Input: part model. Units: mm. Frame: model coordinates. Face numbers are marked on the shaded views. A direction names the side the tool comes from. Coordinates: 2 decimals unless noted, no trailing zeros. Write each loop counter-clockwise with the first axis right and the second up, starting at its lowest first coordinate (ties: lowest second). Pieces come first, ordered by that corner, then holes.
from build123d import *

# Parameters (mm, degrees)
SKETCH1_W           = 100.2
SKETCH1_H           = 54.5
SKETCH1_W_2         = 80.2
SKETCH1_H_2         = 34.5
BOSS_EXTRUDE1_DEPTH = 11.5
CUT_EXTRUDE1_REACH  = 106.474
SKETCH2_R           = 2.6
CUT_EXTRUDE2_REACH  = 76.917
SKETCH3_R           = 5.65
CUT_EXTRUDE3_START  = -2.5
CUT_EXTRUDE3_DEPTH  = 85.2
SKETCH5_R           = 5.65
CUT_EXTRUDE4_DEPTH  = 10
SKETCH6_W           = 26.2
SKETCH6_H           = 8.04
BOSS_EXTRUDE2_DEPTH = 11.5
SKETCH8_R           = 1.8
BOSS_EXTRUDE3_DEPTH = 1
CUT_EXTRUDE5_REACH  = 94.199
SKETCH9_R           = 1.5
CUT_EXTRUDE6_DEPTH  = 2.5
CUT_EXTRUDE7_START  = -5
SKETCH11_R          = 5.65
CUT_EXTRUDE7_DEPTH  = 5
CUT_EXTRUDE9_REACH  = 84.477
SKETCH12_R          = 5.65
SKETCH12_W          = 5.3
SKETCH12_H          = 6.51001002
FILLET1_R           = 1
BOSS_EXTRUDE5_START = 2
SKETCH13_W          = 13.3
SKETCH13_H          = 23
SKETCH13_R          = 5.65
BOSS_EXTRUDE5_DEPTH = 2
CUT_EXTRUDE10_START = -0.5
CUT_EXTRUDE10_DEPTH = 0.5
CUT_EXTRUDE11_DEPTH = 5


with BuildPart() as part:
    # Sketch1 → Boss-Extrude1 (new, symmetric)
    with BuildSketch(Plane(origin=(0, 0, 0), x_dir=(1, 0, 0), z_dir=(0, 1, 0))):
        Rectangle(SKETCH1_W, SKETCH1_H)
        Rectangle(SKETCH1_W_2, SKETCH1_H_2, mode=Mode.SUBTRACT)
    extrude(amount=BOSS_EXTRUDE1_DEPTH, both=True)

    # Cut-Extrude1: up to this face of the body (flat: up to its plane)
    cut_extrude1_end = Plane(part.part.faces().sort_by_distance((-50.1, 0, 0))[0])
    # Sketch2 → Cut-Extrude1 (cut, up to the picked face)
    with BuildSketch(Plane(origin=(50.1, 0, 0), x_dir=(0, 0, -1), z_dir=(1, 0, 0)), mode=Mode.PRIVATE) as cut_extrude1_sk1:
        Circle(SKETCH2_R)
    cut_extrude1_tool1 = split(extrude(cut_extrude1_sk1.sketch, amount=-CUT_EXTRUDE1_REACH, mode=Mode.PRIVATE), bisect_by=cut_extrude1_end, keep=Keep.BOTH, mode=Mode.PRIVATE)
    add(cut_extrude1_tool1.solids().sort_by(Axis((50.1, 0, 0), (-1, 0, 0)))[0], mode=Mode.SUBTRACT)

    # Cut-Extrude2: up to this face of the body (flat: up to its plane)
    cut_extrude2_end = Plane(part.part.faces().sort_by_distance((0, 0, 27.25))[0])
    # Sketch3 → Cut-Extrude2 (cut, up to the picked face)
    with BuildSketch(Plane(origin=(0, 0, -27.25), x_dir=(-1, 0, 0), z_dir=(0, 0, -1)), mode=Mode.PRIVATE) as cut_extrude2_sk1:
        with Locations((-6.6, 0)):
            Circle(SKETCH3_R)
    cut_extrude2_tool1 = split(extrude(cut_extrude2_sk1.sketch, amount=-CUT_EXTRUDE2_REACH, mode=Mode.PRIVATE), bisect_by=cut_extrude2_end, keep=Keep.BOTH, mode=Mode.PRIVATE)
    add(cut_extrude2_tool1.solids().sort_by(Axis((6.6, 0, -27.25), (0, 0, 1)))[0], mode=Mode.SUBTRACT)

    # Sketch4 → Cut-Extrude3 (cut)
    with BuildSketch(Plane.ZY.offset(-40.1).offset(CUT_EXTRUDE3_START)):
        with BuildLine():
            ThreePointArc((1.838477631, -1.838477631), (-3e-09, -2.6), (-1.838477635, -1.838477627))
            Line((-1.838477635, -1.838477627), (0, -3.676955262))
            Line((0, -3.676955262), (1.838477631, -1.838477631))
        make_face()
        with BuildLine():
            ThreePointArc((-1.838477635, -1.838477627), (-2.6, 3e-09), (-1.83847763, 1.838477632))
            Line((-1.83847763, 1.838477632), (-3.676955262, 0))
            Line((-3.676955262, 0), (-1.838477635, -1.838477627))
        make_face()
        with BuildLine():
            Line((1.838477625, 1.838477637), (0, 3.676955262))
            Line((0, 3.676955262), (-1.83847763, 1.838477632))
            ThreePointArc((-1.83847763, 1.838477632), (-4e-09, 2.6), (1.838477625, 1.838477637))
        make_face()
        with BuildLine():
            Line((3.676955262, 0), (1.838477625, 1.838477637))
            ThreePointArc((1.838477625, 1.838477637), (2.402086783, 0.994976928), (2.6, 0))
            ThreePointArc((2.6, 0), (2.402086785, -0.994976924), (1.838477631, -1.838477631))
            Line((1.838477631, -1.838477631), (3.676955262, 0))
        make_face()
    extrude(amount=CUT_EXTRUDE3_DEPTH, mode=Mode.SUBTRACT)

    # Sketch5 → Cut-Extrude4 (cut)
    with BuildSketch(Plane.XY.offset(-27.25)):
        with Locations((-31.9, 0)):
            Circle(SKETCH5_R)
    extrude(amount=CUT_EXTRUDE4_DEPTH, mode=Mode.SUBTRACT)

    # Sketch6 → Boss-Extrude2 (add, symmetric)
    with BuildSketch(Plane(origin=(0, 0, 0), x_dir=(1, 0, 0), z_dir=(0, 1, 0))):
        Polygon((-16.9, 55.29), (-50.1, 55.29), (-50.1, 27.25), (-45.1, 27.25), (-45.1, 37.25), (42.6, 37.25), (42.6, 27.25), (45.1, 27.25), (45.1, 42.25), (-16.9, 42.25), align=None)
        with Locations((-32, 46.27)):
            Rectangle(SKETCH6_W, SKETCH6_H, mode=Mode.SUBTRACT)
    extrude(amount=BOSS_EXTRUDE2_DEPTH, both=True)

    # Sketch8 → Boss-Extrude3 (add)
    with BuildSketch(Plane.XY.offset(-50.29)):
        with Locations((-39.9, 8)):
            Circle(SKETCH8_R)
        with Locations((-23.9, 8)):
            Circle(SKETCH8_R)
        with Locations((-23.9, -8)):
            Circle(SKETCH8_R)
        with Locations((-39.9, -8)):
            Circle(SKETCH8_R)
    extrude(amount=BOSS_EXTRUDE3_DEPTH)

    # Sketch9 → Cut-Extrude5 (cut, up to next)
    with BuildSketch(Plane.XY.offset(-49.29), mode=Mode.PRIVATE) as cut_extrude5_sk1:
        with Locations((-39.9, 8)):
            Circle(SKETCH9_R)
    cut_extrude5_tool1 = extrude(cut_extrude5_sk1.sketch, amount=-CUT_EXTRUDE5_REACH, mode=Mode.PRIVATE) & part.part
    # Sketch9 → Cut-Extrude5 (cut, up to next)
    with BuildSketch(Plane.XY.offset(-49.29), mode=Mode.PRIVATE) as cut_extrude5_sk2:
        with Locations((-23.9, 8)):
            Circle(SKETCH9_R)
    cut_extrude5_tool2 = extrude(cut_extrude5_sk2.sketch, amount=-CUT_EXTRUDE5_REACH, mode=Mode.PRIVATE) & part.part
    # Sketch9 → Cut-Extrude5 (cut, up to next)
    with BuildSketch(Plane.XY.offset(-49.29), mode=Mode.PRIVATE) as cut_extrude5_sk3:
        with Locations((-23.9, -8)):
            Circle(SKETCH9_R)
    cut_extrude5_tool3 = extrude(cut_extrude5_sk3.sketch, amount=-CUT_EXTRUDE5_REACH, mode=Mode.PRIVATE) & part.part
    # Sketch9 → Cut-Extrude5 (cut, up to next)
    with BuildSketch(Plane.XY.offset(-49.29), mode=Mode.PRIVATE) as cut_extrude5_sk4:
        with Locations((-39.9, -8)):
            Circle(SKETCH9_R)
    cut_extrude5_tool4 = extrude(cut_extrude5_sk4.sketch, amount=-CUT_EXTRUDE5_REACH, mode=Mode.PRIVATE) & part.part
    add(cut_extrude5_tool1.solids().sort_by_distance((-39.9, 8, -49.29))[0], mode=Mode.SUBTRACT)
    add(cut_extrude5_tool2.solids().sort_by_distance((-23.9, 8, -49.29))[0], mode=Mode.SUBTRACT)
    add(cut_extrude5_tool3.solids().sort_by_distance((-23.9, -8, -49.29))[0], mode=Mode.SUBTRACT)
    add(cut_extrude5_tool4.solids().sort_by_distance((-39.9, -8, -49.29))[0], mode=Mode.SUBTRACT)

    # Sketch10 → Cut-Extrude6 (cut)
    with BuildSketch(Plane(origin=(0, 0, -55.29), x_dir=(-1, 0, 0), z_dir=(0, 0, -1))):
        Polygon((26.7, 6.383419246), (26.7, 9.616580754), (23.9, 11.233161507), (21.1, 9.616580754), (21.1, 6.383419246), (23.9, 4.766838493), align=None)
        Polygon((42.7, 6.383419246), (42.7, 9.616580754), (39.9, 11.233161507), (37.1, 9.616580754), (37.1, 6.383419246), (39.9, 4.766838493), align=None)
        Polygon((42.7, -9.616580754), (42.7, -6.383419246), (39.9, -4.766838493), (37.1, -6.383419246), (37.1, -9.616580754), (39.9, -11.233161507), align=None)
        Polygon((26.7, -9.616580754), (26.7, -6.383419246), (23.9, -4.766838493), (21.1, -6.383419246), (21.1, -9.616580754), (23.9, -11.233161507), align=None)
    extrude(amount=-CUT_EXTRUDE6_DEPTH, mode=Mode.SUBTRACT)

    # Sketch11 → Cut-Extrude7 (cut)
    with BuildSketch(Plane.XY.offset(-37.25).offset(CUT_EXTRUDE7_START)):
        with Locations((-31.9, 0)):
            Circle(SKETCH11_R)
    extrude(amount=CUT_EXTRUDE7_DEPTH, mode=Mode.SUBTRACT)

    # Sketch12 → Cut-Extrude9 (cut, up to next)
    with BuildSketch(Plane.XY.offset(-37.25), mode=Mode.PRIVATE) as cut_extrude9_sk1:
        with Locations(Location((6.6, 0, 0), (0, 0, 180))):
            Circle(SKETCH12_R)
    cut_extrude9_tool1 = extrude(cut_extrude9_sk1.sketch, amount=-CUT_EXTRUDE9_REACH, mode=Mode.PRIVATE) & part.part
    # Sketch12 → Cut-Extrude9 (cut, up to next)
    with BuildSketch(Plane.XY.offset(-37.25), mode=Mode.PRIVATE) as cut_extrude9_sk2:
        with Locations((6.6, 8.24499499)):
            Rectangle(SKETCH12_W, SKETCH12_H)
    cut_extrude9_tool2 = extrude(cut_extrude9_sk2.sketch, amount=-CUT_EXTRUDE9_REACH, mode=Mode.PRIVATE) & part.part
    add(cut_extrude9_tool1.solids().sort_by_distance((6.6, 0, -37.25))[0], mode=Mode.SUBTRACT)
    add(cut_extrude9_tool2.solids().sort_by_distance((6.6, 8.244995, -37.25))[0], mode=Mode.SUBTRACT)

    # Fillet1
    # the kernel refuses this fillet: 1 mm, written as the material it takes off along each edge
    with BuildSketch(Plane(origin=(-14.4, 11.5, -55.29), x_dir=(0, -1, 0), z_dir=(-1, 0, 0)), Plane(origin=(-14.4, -11.5, -55.29), x_dir=(0, 0, 1), z_dir=(-1, 0, 0))) as fillet1_piece_1:
        with BuildLine():
            CenterArc((FILLET1_R, FILLET1_R), FILLET1_R, 180, 90)
            Line((0, FILLET1_R), (0, 0))
            Line((0, 0), (FILLET1_R, 0))
        make_face()
    extrude(amount=38.2, mode=Mode.SUBTRACT)

    # Sketch13 → Boss-Extrude5 (add)
    with BuildSketch(Plane(origin=(0, 0, -42.25), x_dir=(-1, 0, 0), z_dir=(0, 0, -1)).offset(BOSS_EXTRUDE5_START)):
        with Locations((-6.6, 0)):
            Rectangle(SKETCH13_W, SKETCH13_H)
        with Locations((-6.6, 0)):
            Circle(SKETCH13_R, mode=Mode.SUBTRACT)
    extrude(amount=-BOSS_EXTRUDE5_DEPTH)

    # Sketch14 → Cut-Extrude10 (cut)
    with BuildSketch(Plane.XY.offset(-42.25).offset(CUT_EXTRUDE10_START)):
        with BuildLine():
            Line((3.95, 11.5), (3.95, 4.98998998))
            ThreePointArc((3.95, 4.98998998), (6.6, 5.65), (9.25, 4.98998998))
            Line((9.25, 4.98998998), (9.25, 11.5))
            Line((9.25, 11.5), (3.95, 11.5))
        make_face()
    extrude(amount=CUT_EXTRUDE10_DEPTH, mode=Mode.SUBTRACT)

    # Sketch15 → Cut-Extrude11 (cut)
    with BuildSketch(Plane(origin=(0, 0, -42.25), x_dir=(-1, 0, 0), z_dir=(0, 0, -1))):
        with BuildLine():
            Line((22.9, 4.5), (24.9, 4.5))
            ThreePointArc((24.9, 4.5), (26.314213562, 5.085786438), (26.9, 6.5))
            Line((26.9, 6.5), (26.9, 11.5))
            Line((26.9, 11.5), (20.9, 11.5))
            Line((20.9, 11.5), (20.9, 6.5))
            ThreePointArc((20.9, 6.5), (21.485786438, 5.085786438), (22.9, 4.5))
        make_face()
        with BuildLine():
            Line((40.9, 4.5), (38.9, 4.5))
            ThreePointArc((38.9, 4.5), (37.485786438, 5.085786438), (36.9, 6.5))
            Line((36.9, 6.5), (36.9, 11.5))
            Line((36.9, 11.5), (42.9, 11.5))
            Line((42.9, 11.5), (42.9, 6.5))
            ThreePointArc((42.9, 6.5), (42.314213562, 5.085786438), (40.9, 4.5))
        make_face()
        with BuildLine():
            Line((40.9, -4.5), (38.9, -4.5))
            ThreePointArc((38.9, -4.5), (37.485786438, -5.085786438), (36.9, -6.5))
            Line((36.9, -6.5), (36.9, -11.5))
            Line((36.9, -11.5), (42.9, -11.5))
            Line((42.9, -11.5), (42.9, -6.5))
            ThreePointArc((42.9, -6.5), (42.314213562, -5.085786438), (40.9, -4.5))
        make_face()
        with BuildLine():
            Line((22.9, -4.5), (24.9, -4.5))
            ThreePointArc((24.9, -4.5), (26.314213562, -5.085786438), (26.9, -6.5))
            Line((26.9, -6.5), (26.9, -11.5))
            Line((26.9, -11.5), (20.9, -11.5))
            Line((20.9, -11.5), (20.9, -6.5))
            ThreePointArc((20.9, -6.5), (21.485786438, -5.085786438), (22.9, -4.5))
        make_face()
    extrude(amount=-CUT_EXTRUDE11_DEPTH, mode=Mode.SUBTRACT)


solid = part.part
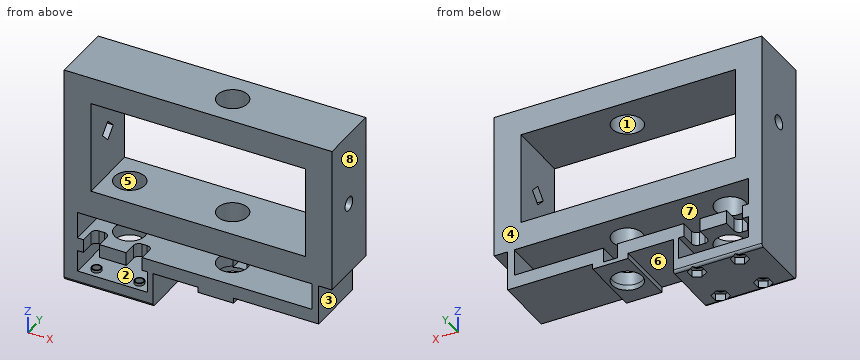
Item 1: Pin query (flat end, axial travel): pin 1 Ø1 at (x, z) = (-23.5, -40.5) entering from +Y; pin 2 Ø2 at (y, z) = (1.5, -33) entering from +X; pin 3 Ø3 at (x, y) = (-7.5, 2.5) entering from -Z. Return the tip coordinate at first contact, or that it passes through.
Item 2: Section query A-A, the plane z = -5.5. Return loops of the section in (x, y), then the cut area to 3 significant figures.
Item 3: Pull-direction query (Y, two-part tool) for the marked faces 1, 2, 3 and 4; classes: released by +Y, released by -Y, zero draft, split by the parting line, or undercut.
Item 4: Access query for the marked faces 5, 6, 7 and 8. Directions: +Z, -Z, +X, -X, +Y, -Y. A direction counts if a zero-diameter tool reaches every point of the face in a straight line with its end or side. Return the directions, or none.
Item 5: Material intervals for line 1 (Z direction, x = -21, y = 4.75); line 2 (Z direction, x = -6.5, y = 3.5); line 3 (X direction, y = 8.25, z = -38.5), sorted ascending.
Item 6: Section query B-B, the plane x = -31.9. Return loops of the section in (y, z), then the cut area to 3 significant figures.
Item 7: Section query C-C, the plane y = -8. State how many separate pieces and enclosed holes the cut face has, then the cut area to 3 significant figures.
Item 8: Section query D-D, the plane x = -2.5. Return loops of the section in (y, z).
The answers:
1. pin 1: stops at y = 4.5
1. pin 2: stops at x = 45.1
1. pin 3: stops at z = -42.25
2. outline: (-50.1, -11.5) - (-40.1, -11.5) - (-40.1, 11.5) - (-50.1, 11.5) - close; (40.1, -11.5) - (50.1, -11.5) - (50.1, 11.5) - (40.1, 11.5) - close
2. area: 460 mm2
3. face 1: undercut
3. face 2: undercut
3. face 3: zero draft
3. face 4: released by +Y
4. face 5: none
4. face 6: -Z, +Y, -Y
4. face 7: +Y, -Y
4. face 8: +Z, -Z, +X, +Y, -Y
5. line 1: z = -55.29 to -50.29, -42.25 to -37.25, -27.25 to -17.25, 17.25 to 27.25
5. line 2: z = -42.25 to -37.25, -27.25 to -17.25, 17.25 to 27.25
5. line 3: x = -50.1 to -42.9, -36.9 to -26.9, -20.9 to 3.95, 9.25 to 45.1
6. outline: (-11.5, -54.29) arc R1 ccw to (-10.5, -55.29) - (10.5, -55.29) arc R1 ccw to (11.5, -54.29) - (11.5, -50.29) - (-11.5, -50.29) - close; (-11.5, -42.25) - (-5.65, -42.25) - (-5.65, -37.25) - (-11.5, -37.25) - close; (-11.5, -27.25) - (-5.65, -27.25) - (-5.65, -17.25) - (-11.5, -17.25) - close; (-11.5, 17.25) - (11.5, 17.25) - (11.5, 27.25) - (-11.5, 27.25) - close; (5.65, -42.25) - (11.5, -42.25) - (11.5, -37.25) - (5.65, -37.25) - close; (5.65, -27.25) - (11.5, -27.25) - (11.5, -17.25) - (5.65, -17.25) - close
6. area: 520 mm2
7. separate pieces: 3
7. enclosed holes: 1
7. area: 3,390 mm2
8. outline: (-11.5, -42.25) - (11.5, -42.25) - (11.5, -37.25) - (-11.5, -37.25) - close; (-11.5, -27.25) - (11.5, -27.25) - (11.5, -17.25) - (-11.5, -17.25) - close; (-11.5, 17.25) - (11.5, 17.25) - (11.5, 27.25) - (-11.5, 27.25) - close
